Autodesk Inventor part; units mm, degrees
ref_plane "YZ Plane" through (0, 0, 0) normal (1, 0, 0) x (0, 1, 0)
ref_plane "XZ Plane" through (0, 0, 0) normal (0, 1, 0) x (-1, 0, 0)
ref_plane "XY Plane" through (0, 0, 0) normal (0, 0, 1) x (1, 0, 0)
sketch "Sketch1" plane through (0, 0, 0) normal (0, 0, 1) x (1, 0, 0)
  circle A0 centre (0, 0) radius 10
  dimension "d0" = 20
extrude "Extrusion1" add sketch "Sketch1" along normal blind 120
sketch "Sketch2" plane through (0, 0, 0) normal (0, 0, -1) x (-1, 0, 0)
  circle A0 centre (0, 0) radius 10
  circle A1 centre (0, 0) radius 5
  dimension "d3" = 10
extrude "Extrusion2" add sketch "Sketch2" along normal blind 20 contours A1
chamfer "Chamfer1" distance 5 distance2 15 1 edges at (5, 0, -20) measured on face at (0.591, 1.5584, -20)
chamfer "Chamfer2" distance 1.5 distance2 32.75 1 edges at (-10, 0, 0) measured on face at (8.188, -1.1966, 0)
fillet "Fillet1" radius 5 1 edges at (-10, 0, 120)
properties part number "Pen"
Geometry check sheet. Reference: the model listing, model coordinates, mm. A direction names the side the tool comes from. Coordinates: 2 decimals unless noted, no trailing zeros. Order: outer loops, then holes, each group sorted by start corner. A loop starts at its lowest first (then second) coordinate and runs counter-clockwise, first axis right, second up. Notation, with made-up numbers: (59, 48.25) - (102, 48.25) arc R36 cw to (102, 82.25) - close; hole circle Ø2 at (53, 32.5). An arc over 180 degrees is marked (long way). Answer as a JSON object with one key per item and string values. Group by question number.
Item 1: Sectioned sample at B-B, the plane z = -2. Record the cut outline in (x, y), and give its area (3 significant figures).
Item 2: Tool access check on faces 1 (the face through (1.08, 4.88, -2.46)), 2 (the face through (-2.17, 9.76, 73.3)). Record the directions out of +Z, -Z, +X, -X, +Y, -Y that give a thin tool (end or side, any length) a straight path to the whole face; none if there is none.
Item 3: Depth check by flat-ended pin: pin 1 Ø12 at (x, z) = (3, -3) entering from +Y; pin 2 Ø12 at (y, z) = (4, 91.5) entering from +X; pin 3 Ø2 at (y, z) = (-7, 93) entering from -X; pin 4 Ø5 at (x, z) = (5, -5) entering from -Y. Enter the tip coordinate at first touch or a pass-through.
Item 4: Sectioned sample at A-A, the plane z = 101.5. Record the cut outline in (x, y), and give its area (3 significant figures).
Item 5: Scan lines: probe 1 along Z at (x, y) = (-4.5, -2.75); probe 2 along X at (y, z) = (0.25, 107.5); probe 3 along X at (y, z) = (4, 90.5). Record each from-to range of solid material in increasing order.
Resolved:
{
 "1": {"outline": "circle Ø10 at (0, 0)", "area": "78.5 mm^2"},
 "2": {"face 1": "-Z", "face 2": "+Z, -Z"},
 "3": {"pin 1": "y = 8.6", "pin 2": "x = 10", "pin 3": "x = -8", "pin 4": "y = -4.33"},
 "4": {"outline": "circle Ø20 at (0, 0)", "area": "314 mm^2"},
 "5": {"probe 1": "0 to 119.99", "probe 2": "-10 to 10", "probe 3": "-9.17 to 9.17"}
}
